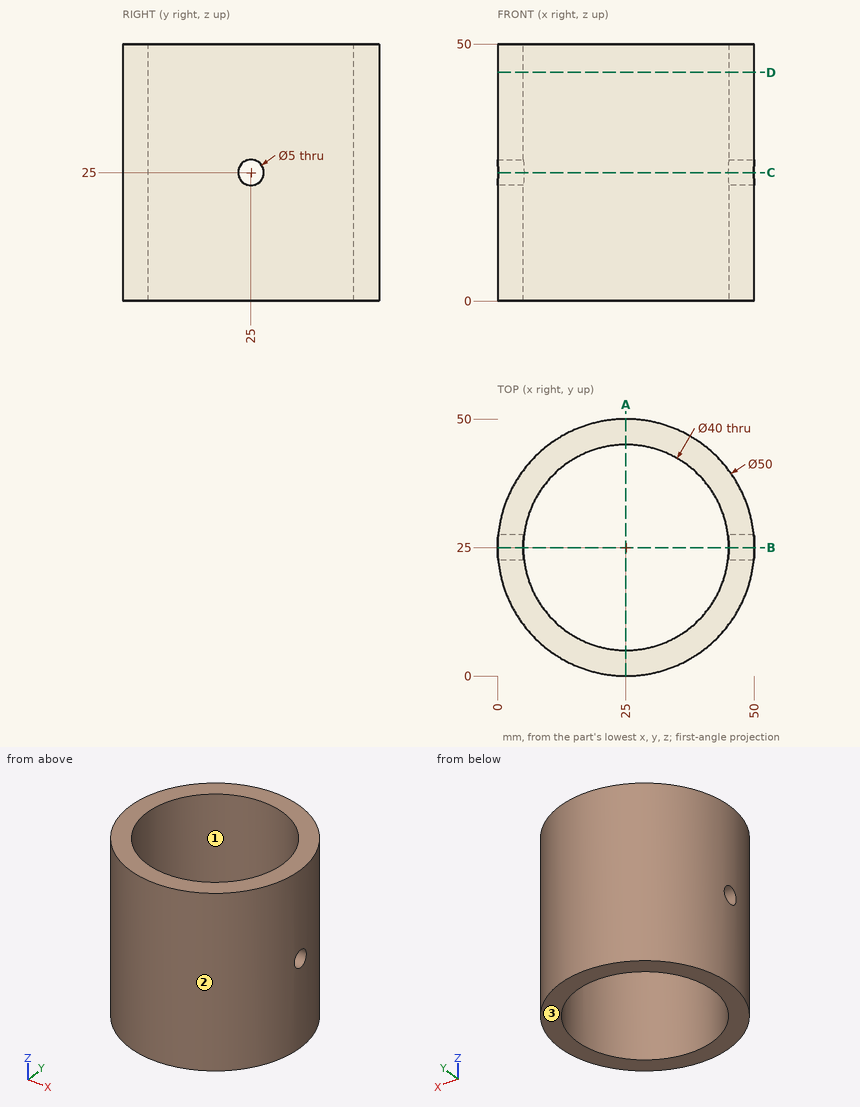
Verification items for this drawing (mm, ordinates from the low corner). Coordinates: 2 decimals unless noted, no trailing zeros. Loops run counter-clockwise (first coordinate to the right, second up) from the corner with the lowest first, then second, coordinate; pieces in that order, holes last. Notation, with made-up numbers: (10.5, 78) - (45.5, 78) arc R31 cw to (45.5, 117) - close; hole circle Ø3 at (9.25, 31.5). An arc over 180 degrees is marked (long way). One line per item, written item: value. Start each with the question number.
(1) Cross-section at D-D on z = 44.5. Enter the section's corners in (x, y), plus the area to 3 significant figures.
(2) Material ranges on line 1 (Y direction, x = 25, z = 15); line 2 (X direction, y = 34.5, z = 8); line 3 (Y direction, x = 27, z = 19), recorded low to high. Write a range as [from, to].
(3) Cross-section at A-A on x = 25. Enter the section's corners in (y, z), plus the area to 3 significant figures.
(4) Cross-section at B-B on y = 25. Enter the section's corners in (x, z), plus the area to 3 significant figures.
(5) Cross-section at C-C on z = 25. Enter the section's corners in (x, y).
(6) Depth check by flat-ended pin: P1, Ø6, axis at x = 11, z = 38, coming from the -Y side; P2, Ø3, axis at x = 36.5, z = 20.5, coming from the +Y side; P3, Ø1, axis at x = 18, z = 34.5, coming from the +Y side. Enter the tip coordinate at first touch or a pass-through.
(7) Mould release check, pull along Y, two halves, no side actions. Record for the marked faces 1, 2 and 3: released by +Y, released by -Y, zero draft, split by the parting line, or undercut.
Results below:
1. outline: circle Ø50 at (25, 25); hole circle Ø40 at (25, 25)
1. area: 707 mm2
2. line 1: y = [0, 5], [45, 50]
2. line 2: x = [1.88, 7.4], [42.6, 48.12]
2. line 3: y = [0.08, 5.1], [44.9, 49.92]
3. outline: (0, 0) - (5, 0) - (5, 50) - (0, 50) - close; (45, 0) - (50, 0) - (50, 50) - (45, 50) - close
3. area: 500 mm2
4. outline: (0, 0) - (5, 0) - (5, 22.5) - (0, 22.5) - close; (0, 27.5) - (5, 27.5) - (5, 50) - (0, 50) - close; (45, 0) - (50, 0) - (50, 22.5) - (45, 22.5) - close; (45, 27.5) - (50, 27.5) - (50, 50) - (45, 50) - close
4. area: 450 mm2
5. outline: (0.13, 22.5) arc R25 ccw to (49.87, 22.5) - (44.84, 22.5) arc R20 cw to (5.16, 22.5) - close; (0.13, 27.5) - (5.16, 27.5) arc R20 cw to (44.84, 27.5) - (49.87, 27.5) arc R25 ccw to start
6. P1: stops at y = 2.55
6. P2: stops at y = 47.91
6. P3: stops at y = 49.14
7. face 1: undercut
7. face 2: split by the parting line
7. face 3: zero draft
